Input: part model. Units: mm. Frame: model coordinates. A direction names the side the tool comes from. Coordinates: 2 decimals unless noted, no trailing zeros. Write each question's results on one line, items separated by ' | '. Start each with the question number.
1. First-contact query: pin 1 (2 mm diameter, centred on x = 34.5, z = -26, fed in from +Y); pin 2 (1 mm diameter, centred on x = -20.5, y = 0, fed in from +Z); pin 3 (0.6 mm diameter, centred on y = -0.5, z = 29, fed in from +X); pin 4 (1 mm diameter, centred on y = 0.5, z = -6.5, fed in from +X). Flat tips, straight axial feed; report the tip coordinate or a pass-through.
2. Section query A-A, the plane y = 0.05. Count the separate pieces of the cut face and the enclosed holes in it, and give its area (3 significant figures).
3. Pull-direction query (Z, two-part tool) for faces 3 (the cylindrical face through (28.294, -0.014, -28.813)), 4 (the cylindrical face through (28.813, -0.014, 28.294)), 5 (the flat face through (-25, 0, 1.25)); classes: +Z half, -Z half, draft (parallel to the pull), parting line (faces both ways), or undercut.
4. Set-up query: faces 1 (the cylindrical face through (-8.753, -0.014, -12.358)), 2 (the cylindrical face through (-28.294, -0.014, 28.813)). Return all of +Z, -Z, +X, -X, +Y, -Y with unobstructed straight access to the full face (end or side cutting, diameter ignored); none if empty.
5. Ray query, probe 1 along X at (y, z) = (0.35, 2); probe 2 along X at (y, z) = (-0.35, 40.4); probe 3 along Z at (x, y) = (-25.5, -0.65). Return the intervals inside material, ascending.
```python
from build123d import *

# Parameters (mm, degrees)
SKETCH1_W                      = 32.5
SKETCH1_H                      = 32.5
BOSS_EXTRUDE1_DEPTH            = 1
M2_CLEARANCE_HOLE1_D           = 2.6
M2_CLEARANCE_HOLE1_CSINK_D     = 2.65
M2_CLEARANCE_HOLE1_CSINK_ANGLE = 90
SKETCH7_R                      = 0.8
BOSS_EXTRUDE2_DEPTH            = 2
CIRPATTERN1_COUNT              = 4
BOSS_EXTRUDE3_DEPTH            = 2
CIRPATTERN3_COUNT              = 4
CUT_EXTRUDE2_DEPTH             = 63.752250956
CIRPATTERN4_COUNT              = 4
FILLET2_R                      = 1
CUT_EXTRUDE3_DEPTH             = 63.752250956
CUT_EXTRUDE3_DEPTH_BACK        = 63.752250956
SKETCH15_R                     = 3.554540671
FILLET1_R                      = 3.75


with BuildPart() as part:
    # Sketch1 → Boss-Extrude1 (new, symmetric)
    with BuildSketch(Plane(origin=(0, 0, 0), x_dir=(1, 0, 0), z_dir=(0, 1, 0))):
        Rectangle(SKETCH1_W, SKETCH1_H)
    extrude(amount=BOSS_EXTRUDE1_DEPTH, both=True)

    # M2 Clearance Hole1 (through all)
    with Locations(Plane(origin=(0, 1, 0), x_dir=(1, 0, 0), z_dir=(0, 1, 0))):
        with Locations((-12.5, -12.5), (-12.5, 12.5), (12.5, -12.5), (12.5, 12.5)):
            CounterSinkHole(M2_CLEARANCE_HOLE1_D / 2, M2_CLEARANCE_HOLE1_CSINK_D / 2, counter_sink_angle=M2_CLEARANCE_HOLE1_CSINK_ANGLE)

    # Sketch7 → Boss-Extrude2 (add)
    with BuildSketch(Plane.XZ.offset(1)):
        with BuildLine():
            Line((16.25, -1.25), (33.291291362, -1.25))
            ThreePointArc((33.291291362, -1.25), (44.35, 0), (33.291291362, 1.25))
            Line((33.291291362, 1.25), (16.25, 1.25))
            Line((16.25, 1.25), (16.25, -1.25))
        make_face()
        with Locations(Location((40.4, 2.857883832, 0), (0, 0, 270))):
            Circle(SKETCH7_R, mode=Mode.SUBTRACT)
        with Locations(Location((40.4, -2.857883832, 0), (0, 0, 270))):
            Circle(SKETCH7_R, mode=Mode.SUBTRACT)
        with Locations(Location((35.45, 0, 0), (0, 0, 270))):
            Circle(SKETCH7_R, mode=Mode.SUBTRACT)
    boss_extrude2 = extrude(amount=-BOSS_EXTRUDE2_DEPTH)

    # CirPattern1: Boss-Extrude2 ×4 about axis
    cirpattern1_axis = Axis((0, 0, 0), (0, 1, 0))
    for i in range(1, CIRPATTERN1_COUNT):
        add(boss_extrude2.rotate(cirpattern1_axis, i * 360 / CIRPATTERN1_COUNT))

    # Sketch13 → Boss-Extrude3 (add)
    with BuildSketch(Plane.XZ.offset(1)):
        with BuildLine():
            ThreePointArc((-5.45586778, -37.487658222), (-26.787039891, -26.787039891), (-37.487658222, -5.45586778))
            ThreePointArc((-37.487658222, -5.45586778), (-38.75, -5.6), (-40.012341778, -5.45586778))
            ThreePointArc((-40.012341778, -5.45586778), (-28.554806844, -28.554806844), (-5.45586778, -40.012341778))
            ThreePointArc((-5.45586778, -40.012341778), (-5.6, -38.75), (-5.45586778, -37.487658222))
        make_face()
    boss_extrude3 = extrude(amount=-BOSS_EXTRUDE3_DEPTH)

    # CirPattern3: Boss-Extrude3 ×4 about axis
    cirpattern3_axis = Axis((0, 0, 0), (0, -1, 0))
    for i in range(1, CIRPATTERN3_COUNT):
        add(boss_extrude3.rotate(cirpattern3_axis, i * 360 / CIRPATTERN3_COUNT))

    # Sketch14 → Cut-Extrude2 (cut, symmetric)
    with BuildSketch(Plane(origin=(0, 1, 0), x_dir=(1, 0, 0), z_dir=(0, 1, 0))):
        with BuildLine():
            Line((-14.75, -1.25), (-14.75, -9.5))
            ThreePointArc((-14.75, -9.5), (-12.739903071, -8.757681666), (-10.651475744, -9.237262181))
            Line((-10.651475744, -9.237262181), (-2.664213562, -1.25))
            Line((-2.664213562, -1.25), (-14.75, -1.25))
        make_face()
        with BuildLine():
            Line((-1.25, -14.75), (-1.25, -2.664213562))
            Line((-1.25, -2.664213562), (-9.237262181, -10.651475744))
            ThreePointArc((-9.237262181, -10.651475744), (-8.757681666, -12.739903071), (-9.5, -14.75))
            Line((-9.5, -14.75), (-1.25, -14.75))
        make_face()
    cut_extrude2 = extrude(amount=CUT_EXTRUDE2_DEPTH, both=True, mode=Mode.SUBTRACT)

    # CirPattern4: Cut-Extrude2 ×4 about axis
    cirpattern4_axis = Axis((0, 0, 0), (0, 1, 0))
    for i in range(1, CIRPATTERN4_COUNT):
        add(cut_extrude2.rotate(cirpattern4_axis, i * 360 / CIRPATTERN4_COUNT), mode=Mode.SUBTRACT)

    # Fillet2
    fillet2_edges = [part.edges().sort_by_distance(p)[0] for p in [
        (1.25, 0, 14.75),
        (9.5, 0, 14.75),
        (9.237262181, 0, 10.651475744),
        (1.25, 0, 2.664213562),
        (10.651475744, 0, 9.237262181),
        (14.75, 0, 9.5),
        (14.75, 0, 1.25),
        (2.664213562, 0, 1.25),
        (14.75, 0, -1.25),
        (9.237262181, 0, -10.651475744),
        (1.25, 0, -2.664213562),
        (2.664213562, 0, -1.25),
        (10.651475744, 0, -9.237262181),
        (14.75, 0, -9.5),
        (9.5, 0, -14.75),
        (1.25, 0, -14.75),
        (-10.651475744, 0, 9.237262181),
        (-2.664213562, 0, -1.25),
        (-9.237262181, 0, -10.651475744),
        (-1.25, 0, 14.75),
        (-14.75, 0, 9.5),
        (-14.75, 0, 1.25),
        (-9.237262181, 0, 10.651475744),
        (-9.5, 0, 14.75),
        (-10.651475744, 0, -9.237262181),
        (-1.25, 0, 2.664213562),
        (-2.664213562, 0, 1.25),
        (-1.25, 0, -14.75),
        (-14.75, 0, -1.25),
        (-1.25, 0, -2.664213562),
        (-14.75, 0, -9.5),
        (-9.5, 0, -14.75),
    ]]
    fillet(fillet2_edges, radius=FILLET2_R)

    # Sketch15 → Cut-Extrude3 (cut, two sides: drawn at the far end of the back side and taken through both)
    with BuildSketch(Plane(origin=(0, 1, 0), x_dir=(1, 0, 0), z_dir=(0, 1, 0)).offset(-CUT_EXTRUDE3_DEPTH_BACK)):
        with Locations(Location((0, 0, 0), (0, 0, 270))):
            Circle(SKETCH15_R)
    extrude(amount=CUT_EXTRUDE3_DEPTH + CUT_EXTRUDE3_DEPTH_BACK, mode=Mode.SUBTRACT)

    # Fillet1
    fillet1_edges = [part.edges().sort_by_distance(p)[0] for p in [
        (-16.25, 0, -16.25),
        (16.25, 0, -16.25),
        (16.25, 0, 16.25),
        (-16.25, 0, 16.25),
    ]]
    fillet(fillet1_edges, radius=FILLET1_R)


solid = part.part
```
Answer:
1) pin 1: through | pin 2: z = 35.08 | pin 3: x = 28.41 | pin 4: x = 39.93
2) separate pieces: 1 | enclosed holes: 29 | area: 1,530 mm^2
3) face 3: -Z half | face 4: +Z half | face 5: undercut
4) face 1: +Y, -Y | face 2: +Z, -X, +Y, -Y
5) probe 1: -43.98 to -33.52, -16.25 to -14.72, -4.11 to -2.94, 2.94 to 4.11, 14.72 to 16.25, 33.52 to 43.98 | probe 2: -5.35 to -3.66, -2.06 to 2.06, 3.66 to 5.35 | probe 3: -31.31 to -28.02, -1.25 to 1.25, 28.02 to 31.31
